Check sheet for the modelled part. Datum: model origin and axes. Units: mm. A direction names the side the tool comes from. Round coordinates to 2 decimals unless told otherwise and drop trailing zeros. Write each loop counter-clockwise with the first axis right and the second up, starting at its lowest first coordinate (ties: lowest second). Pieces come first, ordered by that corner, then holes.
Item 1: Release check for a two-part mould opening along Z. For faces 4 (the cylindrical face through (2.213, -2.788, -16.855)), 5 (the cylindrical face through (11.19, -13.58, -0.49)), 6 (the flat face through (-4, 0, 14)) record: pulls with the +Z half, pulls with the -Z half, needs draft (parallel to the pull), parting line crosses it, or undercut.
Item 2: Section check B-B, the plane y = -16.25. Record the cut outline in (x, z), plus the area to 3 significant figures.
Item 3: Material ranges on line 1 along Z through (x, y) = (0, -17.25); line 2 along Z through (x, y) = (-9, -13); line 3 along X through (y, z) = (-15.75, 3), recorded low to high.
Item 4: Section check C-C, the plane y = -6. Record the cut outline in (x, z).
Item 5: Depth check by flat-ended pin: pin 1 (10 mm diameter, centred on x = -1.5, z = -10.5, fed in from -Y); pin 2 (18 mm diameter, centred on x = 0, z = 0, fed in from -Y); pin 3 (6 mm diameter, centred on x = 3.5, y = -4, fed in from +Z); pin 4 (12 mm diameter, centred on x = 3, y = -18, fed in from +Z). Enter the tip coordinate at first touch or a pass-through.
Item 6: Section check A-A, the plane x = 0. Record the cut outline in (y, z).
Item 7: Set-up check for faces 1 (the cylindrical face through (1.85, -2.14, -14.08)), 2 (the cylindrical face through (-12.932, -15.344, 5.362)), 3 (the flat face through (4, -22, -13)): record each of +Z, -Z, +X, -X, +Y, -Y from which the full face is reachable in a straight line by a thin tool's end or side.
from build123d import *

# Parameters (mm, degrees)
CHAMFER1_SIZE = 2


with BuildPart() as part:
    # Sketch1 → Revolve1 (revolve)
    with BuildSketch(Plane.XY, mode=Mode.PRIVATE) as revolve1_sk:
        Polygon((17, 0), (17, -5.5), (14, -8.5), (14, -22), (11.2, -22), (11.2, -7.340202025), (14.2, -4.340202025), (14.2, 0), align=None)
    revolve(revolve1_sk.sketch.rotate(Axis((0, 16.279491968, 0), (0, -1, 0)), 180), axis=Axis((0, 16.279491968, 0), (0, -1, 0)))

    # Chamfer1
    chamfer1_edges = [part.edges().sort_by_distance(p)[0] for p in [
        (11.2, -22, 0),
    ]]
    chamfer(chamfer1_edges, length=CHAMFER1_SIZE)


solid = part.part
Values found:
1. face 4: parting line crosses it
1. face 5: undercut
1. face 6: needs draft
2. outline: circle Ø28 at (0, 0); hole circle Ø22.4 at (0, 0)
2. area: 222 mm2
3. line 1: z = -14 to -11.2, 11.2 to 14
3. line 2: z = -10.72 to -6.67, 6.67 to 10.72
3. line 3: x = -13.67 to -10.79, 10.79 to 13.67
4. outline: circle Ø33 at (0, 0); hole circle Ø25.08 at (0, 0)
5. pin 1: stops at y = -22
5. pin 2: passes through
5. pin 3: stops at z = 16.99
5. pin 4: stops at z = 14
6. outline: (-22, -14) - (-8.5, -14) - (-5.5, -17) - (0, -17) - (0, -14.2) - (-4.34, -14.2) - (-7.34, -11.2) - (-20, -11.2) - (-22, -13.2) - close; (-22, 13.2) - (-20, 11.2) - (-7.34, 11.2) - (-4.34, 14.2) - (0, 14.2) - (0, 17) - (-5.5, 17) - (-8.5, 14) - (-22, 14) - close
7. face 1: +Y
7. face 2: -Y
7. face 3: +Z, -Z, +X, -X, -Y
